Geometry: final body of the model. Coordinates: model frame, mm. A direction names the side the tool comes from. Round coordinates to 2 decimals unless told otherwise and drop trailing zeros. Loops run counter-clockwise (first coordinate to the right, second up) from the corner with the lowest first, then second, coordinate; pieces in that order, holes last. Notation, with made-up numbers: M 4,24 L 34,24 A22 cw 34,57 Z; hole C -36,-26.5 d9. An arc over 180 degrees is marked long. Return JSON: item names as keys, results as strings.
from build123d import *

# Parameters (mm, degrees)
F0_W     = 609.6
F0_H     = 1219.2
F1_DEPTH = 25.4
F2_W     = 558.8
F2_H     = 1168.4
F2_W_2   = 457.2
F2_H_2   = 1066.8
F3_DEPTH = 50.8
F4_W     = 50.8
F4_H     = 50.8
F5_DEPTH = 685.8


with BuildPart() as f1:
    # F0 (on Top) → F1 (new body)
    with BuildSketch(Plane.XY):
        with Locations((-10.056729, -14.887511)):
            Rectangle(F0_W, F0_H)
    extrude(amount=F1_DEPTH)

    # F2 (on face) → F3 (join)
    with BuildSketch(Plane.XY.offset(25.4)):
        with Locations((-10.056729, -14.887511)):
            Rectangle(F2_W, F2_H)
        with Locations((-10.056729, -14.887511)):
            Rectangle(F2_W_2, F2_H_2, mode=Mode.SUBTRACT)
    extrude(amount=F3_DEPTH)

    # F4 (on face) → F5 (join)
    with BuildSketch(Plane.XY.offset(76.2)):
        with Locations((-264.056729, 543.912489)):
            Rectangle(F4_W, F4_H)
        with Locations((243.943271, 543.912489)):
            Rectangle(F4_W, F4_H)
        with Locations((-264.056729, -573.687511)):
            Rectangle(F4_W, F4_H)
        with Locations((243.943271, -573.687511)):
            Rectangle(F4_W, F4_H)
    extrude(amount=F5_DEPTH)


solid = f1.part
Q1. Section query B-B (x = -36.5). Output: boundary loops of the cut face in (y, z), plus the area to 3 significant figures.
Determined:
{"outline": "M -624.49,0 L 594.71,0 L 594.71,25.4 L 569.31,25.4 L 569.31,76.2 L 518.51,76.2 L 518.51,25.4 L -548.29,25.4 L -548.29,76.2 L -599.09,76.2 L -599.09,25.4 L -624.49,25.4 Z", "area": "36,100 mm^2"}
Q2. Section query C-C (y = 161.5). Output: boundary loops of the cut face in (x, z).
Determined:
{"outline": "M -314.86,0 L 294.74,0 L 294.74,25.4 L 269.34,25.4 L 269.34,76.2 L 218.54,76.2 L 218.54,25.4 L -238.66,25.4 L -238.66,76.2 L -289.46,76.2 L -289.46,25.4 L -314.86,25.4 Z"}
Q3. Reachability of faces 1 (the flat face through (-13, -7, 25.4)), 2 (the flat face through (-239, 569.312, 310)), 3 (the flat face through (-264, -548.288, 414)), 4 (the flat face through (-13, 544, 76.2)) from +Z, -Z, +X, -X, +Y, -Y: full face, straight path, thin tool, end or side. Return the list, or none.
Determined:
{"face 1": "+Z", "face 2": "+Z, +X, -X, +Y", "face 3": "+Z, +X, -X", "face 4": "+Z, +Y, -Y"}
Q4. Pull-direction query (X, two-part tool) for faces 5 (the flat face through (294.743, -23, 13)), 6 (the flat face through (-13, -548.288, 50)), 7 (the flat face through (-239, -599.088, 310)); classes: pulls with the +X half, pulls with the -X half, needs draft (parallel to the pull), parting line crosses it, or undercut.
Determined:
{"face 5": "pulls with the +X half", "face 6": "undercut", "face 7": "needs draft"}
Q5. Pin query (flat end, axial travel): pin 1 (15 mm diameter, centred on y = -567, z = 495, fed in from +X); pin 2 (15 mm diameter, centred on y = -568, z = 377.5, fed in from -X); pin 3 (3 mm diameter, centred on x = 226.5, z = 521.5, fed in from -Y). Return the tip coordinate at first contact, or that it passes through.
Determined:
{"pin 1": "stops at x = 269.34", "pin 2": "stops at x = -289.46", "pin 3": "stops at y = -599.09"}
Q6. Section query A-A (z = 546.5). Output: boundary loops of the cut face in (x, y), plus the area to 3 significant figures.
Determined:
{"outline": "M -289.46,-599.09 L -238.66,-599.09 L -238.66,-548.29 L -289.46,-548.29 Z; M -289.46,518.51 L -238.66,518.51 L -238.66,569.31 L -289.46,569.31 Z; M 218.54,-599.09 L 269.34,-599.09 L 269.34,-548.29 L 218.54,-548.29 Z; M 218.54,518.51 L 269.34,518.51 L 269.34,569.31 L 218.54,569.31 Z", "area": "10,300 mm^2"}
Q7. Material intervals for L1, parallel to Y at x = 230.5, z = 431; L2, parallel to Z at x = -125, y = 502.5; L3, parallel to Z at x = 249, y = -135, sorted ascending.
Determined:
{"L1": "y = -599.09 to -548.29, 518.51 to 569.31", "L2": "z = 0 to 25.4", "L3": "z = 0 to 76.2"}
